Verification items for this drawing (mm, ordinates from the low corner). A direction names the side the tool comes from. Coordinates: 2 decimals unless noted, no trailing zeros. Order: outer loops, then holes, each group sorted by start corner. A loop starts at its lowest first (then second) coordinate and runs counter-clockwise, first axis right, second up. Notation, with made-up numbers: M 31.25,81.5 L 52.25,81.5 A31 cw 52.25,116.5 Z; hole C 65,51 d11. An arc over 180 degrees is marked long. Return JSON: item names as keys, results as strings. Group by question number.
1. Material ranges on line 1 along X through (y, z) = (46, 5) (1 decimal); line 2 along Y through (x, z) = (51, 6.5) (1 decimal); line 3 along X through (y, z) = (17, 30) (1 decimal), recorded low to high.
2. Section check C-C, the plane x = 83.5. Record the cut outline in (y, z).
3. Section check B-B, the plane y = 20. Record the cut outline in (x, z) (1 decimal), plus the area to 3 significant figures.
4. Section check D-D, the plane x = 48.5. Record the cut outline in (y, z) (1 decimal).
5. Set-up check for the marked faces 1, 2, 3, 4 and 5: record each of +Z, -Z, +X, -X, +Y, -Y from which the full face is reachable in a straight line by a thin tool's end or side.
6. Section check A-A, the plane z = 10.5. Record the cut outline in (x, y) (1 decimal).
7. Mould release check, pull along X, two halves, no side actions. Record for the marked faces 6, 7 and 8: +X half, -X half, draft (parallel to the pull), parting line (faces both ways), or undercut.
8. Gauge pin test, flat ends, axial feed: pin 1 (2 mm diameter, centred on y = 32, z = 18.5, fed in from -X) (1 decimal); pin 2 (4 mm diameter, centred on y = 67, z = 16.5, fed in from -X); pin 3 (4 mm diameter, centred on x = 35.5, z = 3.5, fed in from -Y). Record the tip position at first contact, or that the pin passes through.
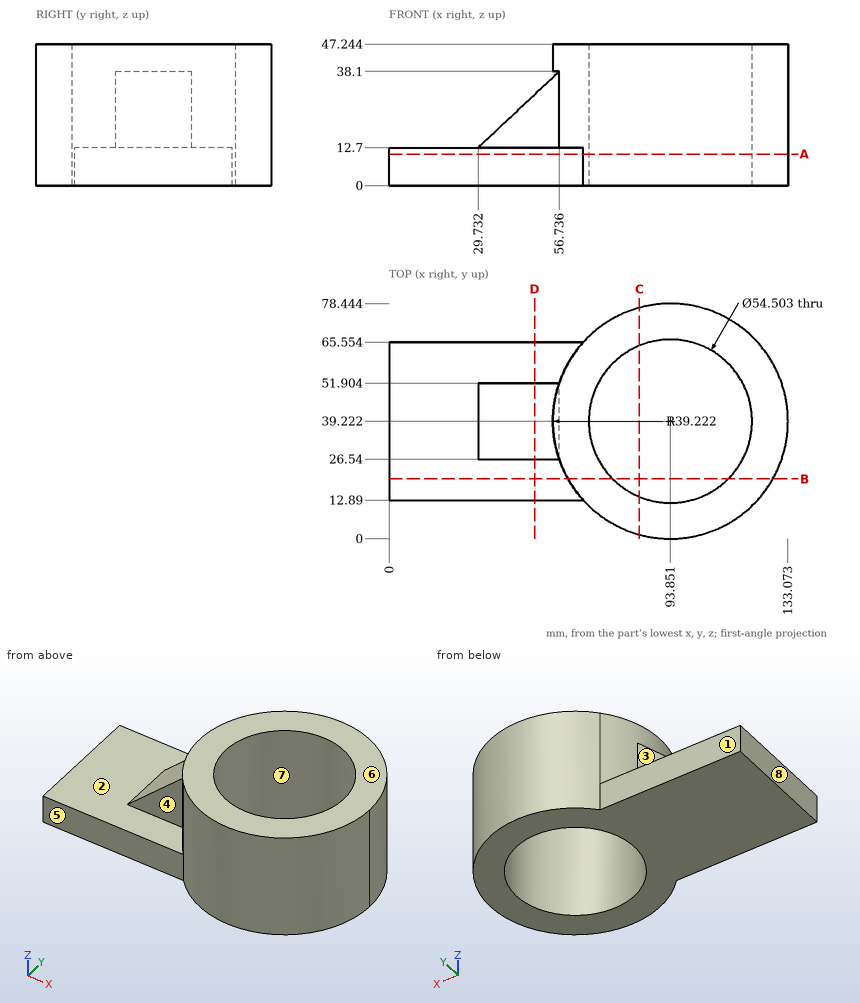
Answers follow:
{
 "1": {"line 1": "0 to 67.5, 120.2 to 132.5", "line 2": "12.9 to 65.6", "line 3": "61.5 to 78.1, 109.6 to 126.2"},
 "2": {"outline": "M 1.39,0 L 14.01,0 L 14.01,47.24 L 1.39,47.24 Z; M 64.43,0 L 77.05,0 L 77.05,47.24 L 64.43,47.24 Z"},
 "3": {"outline": "M 0,0 L 74.5,0 L 74.5,47.2 L 59.7,47.2 L 59.7,12.7 L 0,12.7 Z; M 113.2,0 L 128,0 L 128,47.2 L 113.2,47.2 Z", "area": "2,160 mm^2"},
 "4": {"outline": "M 12.9,0 L 65.6,0 L 65.6,12.7 L 51.9,12.7 L 51.9,30.4 L 26.5,30.4 L 26.5,12.7 L 12.9,12.7 Z"},
 "5": {"face 1": "+Z, -Z, -X, +Y", "face 2": "+Z, -X", "face 3": "+Z, -X, +Y", "face 4": "+Z, -X, -Y", "face 5": "+Z, -Z, -X, -Y"},
 "6": {"outline": "M 0,12.9 L 64.8,12.9 A39.2 ccw 133.1,39.2 A39.2 ccw 64.8,65.6 L 0,65.6 Z; hole C 93.9,39.2 d54.5"},
 "7": {"face 6": "draft", "face 7": "undercut", "face 8": "-X half"},
 "8": {"pin 1": "x = 34.8", "pin 2": "x = 64.29", "pin 3": "y = 12.89"}
}
